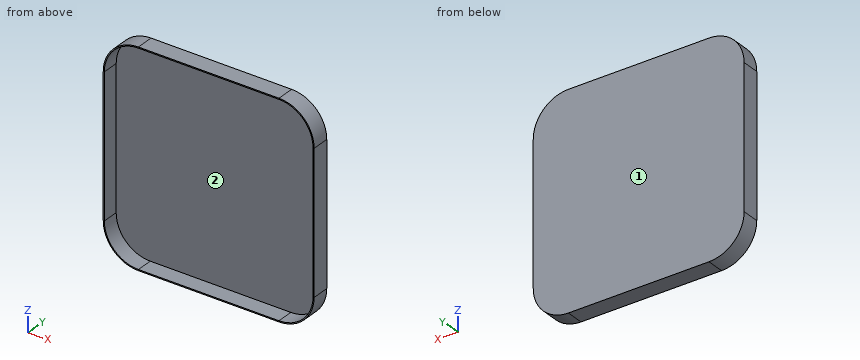
```python
from build123d import *

# Parameters (mm, degrees)
F1_DEPTH = 25.4
F2_T     = -1.6002


with BuildPart() as f1:
    # F0 (on Front) → F1 (new body)
    with BuildSketch(Plane.XZ):
        with BuildLine():
            ThreePointArc((152.4, 101.6), (137.521024, 137.521024), (101.6, 152.4))
            Line((101.6, 152.4), (-101.6, 152.4))
            ThreePointArc((-101.6, 152.4), (-137.521024, 137.521024), (-152.4, 101.6))
            Line((-152.4, 101.6), (-152.4, -101.6))
            ThreePointArc((-152.4, -101.6), (-137.521024, -137.521024), (-101.6, -152.4))
            Line((-101.6, -152.4), (101.6, -152.4))
            ThreePointArc((101.6, -152.4), (137.521024, -137.521024), (152.4, -101.6))
            Line((152.4, -101.6), (152.4, 101.6))
        make_face()
    extrude(amount=F1_DEPTH)

    # F2
    f2_openings = [f1.faces().sort_by_distance(p)[0] for p in [
        (0, -25.4, 0),
    ]]
    offset(amount=F2_T, openings=f2_openings)


solid = f1.part
```
Here's how the part is built. I have some questions about the finished solid (model axes, mm). Face numbers are marked on the shaded views. Coordinates: 2 decimals unless noted, no trailing zeros. Loops run counter-clockwise (first coordinate to the right, second up) from the corner with the lowest first, then second, coordinate; pieces in that order, holes last. Notation, with made-up numbers: M 57.5,-18 L 107.5,-18 A24 ccw 107.5,0 Z; hole C 30,15.25 d3. An arc over 180 degrees is marked long. One line per item, written item: value.
1. Please list where these lines run through material, in increasing order: probe 1 along Z at (x, y) = (-68, -20); probe 2 along Y at (x, z) = (81, 70).
Geometry says:
probe 1: z = -152.4 to -150.8, 150.8 to 152.4
probe 2: y = -1.6 to 0
2. Thinking about a two-plate mould opening in X: for the marked faces 1 and 2, which applies, +X half, -X half, draft (parallel to the pull), parting line (faces both ways), or undercut?
Geometry says:
face 1: draft
face 2: undercut
3. Imagine slicing it at B-B (x = 34). List the corners of the cut face in (y, z) for me, and give its area (3 significant figures).
Geometry says:
outline: M -25.4,-152.4 L 0,-152.4 L 0,152.4 L -25.4,152.4 L -25.4,150.8 L -1.6,150.8 L -1.6,-150.8 L -25.4,-150.8 Z
area: 564 mm2
4. Will these pins go through, and if not, where does the flat tip stop? pin 1 Ø1.5 at (x, z) = (56.5, -58) entering from -Y; pin 2 Ø5 at (x, y) = (108, -11.5) entering from +Z; pin 3 Ø5 at (y, z) = (-20, -105.5) entering from -X.
Geometry says:
pin 1: stops at y = -1.6
pin 2: stops at z = 152.25
pin 3: stops at x = -152.38
5. Imagine slicing it at A-A (y = -15.75). List the corners of the cut face in (x, z) for me.
Geometry says:
outline: M -152.4,-101.6 A50.8 ccw -101.6,-152.4 L 101.6,-152.4 A50.8 ccw 152.4,-101.6 L 152.4,101.6 A50.8 ccw 101.6,152.4 L -101.6,152.4 A50.8 ccw -152.4,101.6 Z; hole M -150.8,-101.6 A49.2 ccw -101.6,-150.8 L 101.6,-150.8 A49.2 ccw 150.8,-101.6 L 150.8,101.6 A49.2 ccw 101.6,150.8 L -101.6,150.8 A49.2 ccw -150.8,101.6 Z
6. Imagine slicing it at C-C (z = 55). List the corners of the cut face in (x, y) for me.
Geometry says:
outline: M -152.4,-25.4 L -150.8,-25.4 L -150.8,-1.6 L 150.8,-1.6 L 150.8,-25.4 L 152.4,-25.4 L 152.4,0 L -152.4,0 Z
